Verification items for the finished model (mm, model axes). Face numbers are marked on the shaded views. Give positions to 0.01 mm unless a question says otherwise; leave off trailing zeros. Order: outer loops, then holes, each group sorted by start corner. A loop starts at its lowest first (then second) coordinate and runs counter-clockwise, first axis right, second up.
(1) Scan lines: L1, parallel to Z at x = -37, y = 1.25 (3 decimals); L2, parallel to Z at x = -10, y = 2.75 (3 decimals); L3, parallel to X at y = 4.75, z = -160. Record each from-to range of solid material in increasing order.
(2) Sectioned sample at B-B on z = -43. Record the cut outline in (x, y), plus the area to 3 significant figures.
(3) Gauge pin test, flat ends, axial feed: pin 1 (4 mm diameter, centred on x = -58, y = 2, fed in from +Z); pin 2 (4 mm diameter, centred on x = -115.5, y = 4.5, fed in from -Z); pin 3 (10 mm diameter, centred on x = -24.5, z = -106.5, fed in from +Y); pin 4 (2 mm diameter, centred on x = -6, z = -34.075, fed in from -Y). Record the tip position at first contact, or that the pin passes through.
(4) Mould release check, pull along Z, two halves, no side actions. Record for the marked faces 1 and 2: pulls with the +Z half, pulls with the -Z half, needs draft (parallel to the pull), parting line crosses it, or undercut.
(5) Sectioned sample at A-A on x = -75.5. Record the cut outline in (y, z) (3 decimals).
(6) Sectioned sample at C-C on y = 6.5. Count the separate pieces of the cut face and the enclosed holes in it, plus the area to 3 significant figures.
Autodesk Inventor part; units mm, degrees
ref_plane "YZ Plane" through (0, 0, 0) normal (1, 0, 0) x (0, 1, 0)
ref_plane "XZ Plane" through (0, 0, 0) normal (0, 1, 0) x (-1, 0, 0)
ref_plane "XY Plane" through (0, 0, 0) normal (0, 0, 1) x (1, 0, 0)
sketch "Base Sketch" plane through (0, 0, 0) normal (0, 1, 0) x (-1, 0, 0)
  line L0 (10, 0) -> (110, 0)
  line L1 (120, -10) -> (120, -160)
  line L2 (110, -170) -> (10, -170)
  line L3 (0, -160) -> (0, -10)
  line L4 (86.3, -30.165) -> (2, -30.165) construction
  line L5 (2, -30.165) -> (2, -139.835) construction
  line L6 (2, -139.835) -> (86.3, -139.835) construction
  line L7 (86.3, -139.835) -> (86.3, -30.165) construction
  line L8 (82.3, -34.075) -> (6, -34.075) construction
  line L9 (6, -34.075) -> (6, -135.925) construction
  line L10 (6, -135.925) -> (82.3, -135.925) construction
  line L11 (82.3, -135.925) -> (82.3, -34.075) construction
  line L12 (0, -10) -> (10, 0)
  line L13 (120, -10) -> (110, 0)
  line L14 (120, -160) -> (110, -170)
  line L15 (0, -160) -> (10, -170)
  line L16 (100, 0) -> (100, -10)
  line L17 (120, -20) -> (110, -20)
  line L18 (100, -10) -> (110, -20)
  line L19 (120, -85) -> (0, -85) construction
  line L20 (60, 0) -> (60, -170) construction
  line L21 (100, -170) -> (100, -160)
  line L22 (120, -150) -> (110, -150)
  line L23 (100, -160) -> (110, -150)
  line L24 (20, 0) -> (20, -10)
  line L25 (0, -20) -> (10, -20)
  line L26 (20, -10) -> (10, -20)
  line L27 (20, -170) -> (20, -160)
  line L28 (20, -160) -> (10, -150)
  line L29 (0, -150) -> (10, -150)
  circle A0 centre (82.3, -34.075) radius 3
  circle A1 centre (6, -34.075) radius 3
  circle A2 centre (82.3, -135.925) radius 3
  circle A3 centre (6, -135.925) radius 3
  line L30 (82.8, -5) -> (82.8, -31.117)
  line L31 (80.3, -5) -> (80.3, -31.8389)
  line L32 (80.3, -36.3111) -> (80.3, -133.6889)
  line L33 (80.3, -138.1611) -> (80.3, -165)
  line L34 (82.8, -37.033) -> (82.8, -132.967)
  line L35 (82.8, -138.883) -> (82.8, -165)
  line L36 (79.5728, -35.325) -> (8.7272, -35.325)
  line L37 (79.5728, -32.825) -> (8.7272, -32.825)
  line L38 (85.0272, -35.325) -> (115, -35.325)
  line L39 (85.0272, -32.825) -> (115, -32.825)
  line L40 (8.7272, -134.675) -> (79.5728, -134.675)
  line L41 (85.0272, -134.675) -> (115, -134.675)
  line L42 (8.7272, -137.175) -> (79.5728, -137.175)
  line L43 (85.0272, -137.175) -> (115, -137.175)
  line L44 (80.3, -165) -> (12.0711, -165)
  line L45 (12.0711, -165) -> (5, -157.9289)
  line L46 (5, -157.9289) -> (5, -12.0711)
  line L47 (5, -12.0711) -> (12.0711, -5)
  line L48 (12.0711, -5) -> (80.3, -5)
  line L49 (82.8, -165) -> (107.9289, -165)
  line L50 (107.9289, -165) -> (115, -157.9289)
  line L51 (115, -157.9289) -> (115, -137.175)
  line L52 (82.8, -5) -> (107.9289, -5)
  line L53 (107.9289, -5) -> (115, -12.0711)
  line L54 (115, -12.0711) -> (115, -32.825)
  line L55 (115, -134.675) -> (115, -35.325)
  point P0 (0, 0)
  point P1 (120, -170)
  point P2 (120, 0)
  point P3 (0, -170)
  point P4 (110, -10)
  point P5 (110, -160)
  point P6 (10, -10)
  point P7 (10, -160)
  point P8 (20, -165)
  point P9 (100, -165)
  point P10 (115, -150)
  point P11 (115, -20)
  point P12 (100, -5)
  point P13 (20, -5)
  point P14 (5, -150)
  point P15 (5, -138.7534)
  point P16 (5, -133.0966)
  point P17 (5, -36.9034)
  point P18 (5, -31.2466)
  point P19 (5, -20)
  dimension "d109" = 6
  dimension "d0" = 120
  dimension "d1" = 170
  dimension "d12" = 84.3
  dimension "d13" = 109.67
  dimension "d14" = 76.3
  dimension "d15" = 101.85
  dimension "d16" = 3.91
  dimension "d17" = 3.91
  dimension "d18" = 4
  dimension "d19" = 4
  dimension "d20" = 2
  dimension "d21" = 30.165
  dimension "d22" = 30.165
  dimension "d82" = 10
  dimension "d83" = 10
  dimension "d84" = 10
  dimension "d85" = 10
  dimension "d88" = 10
  dimension "d90" = 10
  dimension "d91" = 10
  dimension "d93" = 10
  dimension "d94" = 190.9188
  dimension "d95" = 10
  dimension "d96" = 0
  dimension "d101" = 10
  dimension "d102" = 10
  dimension "d103" = 10
  dimension "d104" = 10
  dimension "d113" = 76.3
  dimension "d116" = 101.85
  dimension "d143" = 10
  dimension "d144" = 10
  dimension "d166" = 90
  dimension "d167" = 90
  dimension "d168" = 90
  dimension "d169" = 90
  dimension "d170" = 90
  dimension "d171" = 135
  dimension "d172" = 135
  dimension "d173" = 45
  dimension "d174" = 45
  dimension "d175" = 45
  dimension "d176" = 45
  dimension "d177" = 5
  dimension "d178" = 37.2
  dimension "d179" = 39.7
  dimension "d180" = 115
  dimension "d181" = 5
  dimension "d182" = 185.9188
  dimension "d183" = 9.1421
  dimension "d184" = 180.9188
  dimension "d185" = 2.5
  dimension "d186" = 104.35
  dimension "d187" = 101.85
  dimension "d188" = 27.825
  dimension "d189" = 132.175
  dimension "d190" = 12.825
  dimension "d191" = 160
  dimension "d192" = 115
  dimension "d193" = 115
  dimension "d194" = 82.8
  dimension "d195" = 82.8
  dimension "d196" = 80.3
  dimension "d197" = 80.3
extrude "Main Body" add sketch "Base Sketch" against normal blind 1.5
extrude "Structure" add sketch "Base Sketch" along normal blind 3.5 contours L0 L16 L52 L30 A0 L31 L48 L24 | L25 L46 A1 A3 L29 L3 | L1 L22 L51 L43 A2 L41 L55 L38 A0 L39 L54 L17 | A0 L36 A1 L37 | L27 L44 L33 A2 L35 L49 L21 L2 | A3 L40 A2 L42 | A0 L34 A2 L32
extrude "Corners" add sketch "Base Sketch" along normal blind 8.5 contours L0 L24 L48 L47 L46 L25 L3 L12 | L0 L13 L1 L17 L54 L53 L52 L16 | L24 L26 L25 L46 L47 L48 | L52 L53 L54 L17 L18 L16 | L29 L46 L45 L44 L27 L2 L15 L3 | L29 L28 L27 L44 L45 L46 | L1 L14 L2 L21 L49 L50 L51 L22 | L51 L50 L49 L21 L23 L22
extrude "Board Standoffs" add sketch "Base Sketch" along normal blind 13 contours A0 | L46 A1 | A1 L46 | L46 A3 | A3 L46 | A2
hole "Standoff Hole" at (-6, 0, -34.075) at (-6, 0, -135.925) at (-82.3, 0, -135.925) at (-82.3, 0, -34.075) direction (0, -1, 0) diameter 2.5 end through all both
hole "Corner Hole" at (-110, 0, -10) at (-110, 0, -160) at (-10, 0, -10) at (-10, 0, -160) direction (0, -1, 0) diameter 4.5 end through all both
equation "\"d16\" = d17"
equation "\"d18\" = d19"
equation "\"d21\" = d22"
properties part number "Prod5.2.1 - SKR1.4 Turbo Case Base"
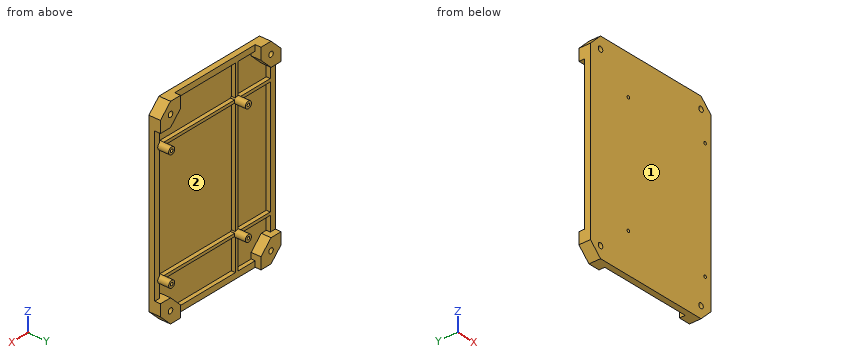
Ans:
1. L1: z = -170 to -165, -137.175 to -134.675, -35.325 to -32.825, -5 to 0
1. L2: z = -170 to -162.25, -157.75 to -150, -137.175 to -134.675, -35.325 to -32.825, -20 to -12.25, -7.75 to 0
1. L3: x = -120 to -112.25, -107.75 to -100, -20 to -12.25, -7.75 to 0
2. outline: (-120, -1.5) - (0, -1.5) - (0, 3.5) - (-5, 3.5) - (-5, 0) - (-80.3, 0) - (-80.3, 3.5) - (-82.8, 3.5) - (-82.8, 0) - (-115, 0) - (-115, 3.5) - (-120, 3.5) - close
2. area: 224 mm2
3. pin 1: stops at z = 0
3. pin 2: stops at z = -166.5
3. pin 3: stops at y = 0
3. pin 4: passes through
4. face 1: needs draft
4. face 2: undercut
5. outline: (-1.5, -170) - (3.5, -170) - (3.5, -165) - (0, -165) - (0, -137.175) - (3.5, -137.175) - (3.5, -134.675) - (0, -134.675) - (0, -35.325) - (3.5, -35.325) - (3.5, -32.825) - (0, -32.825) - (0, -5) - (3.5, -5) - (3.5, 0) - (-1.5, 0) - close
6. separate pieces: 8
6. enclosed holes: 8
6. area: 1,230 mm2
